Job drawing, mm, ordinate dimensions from the low corner. One solid piece. A direction names the side the tool comes from. Round coordinates to 2 decimals unless told otherwise and drop trailing zeros. Loops run counter-clockwise (first coordinate to the right, second up) from the corner with the lowest first, then second, coordinate; pieces in that order, holes last.
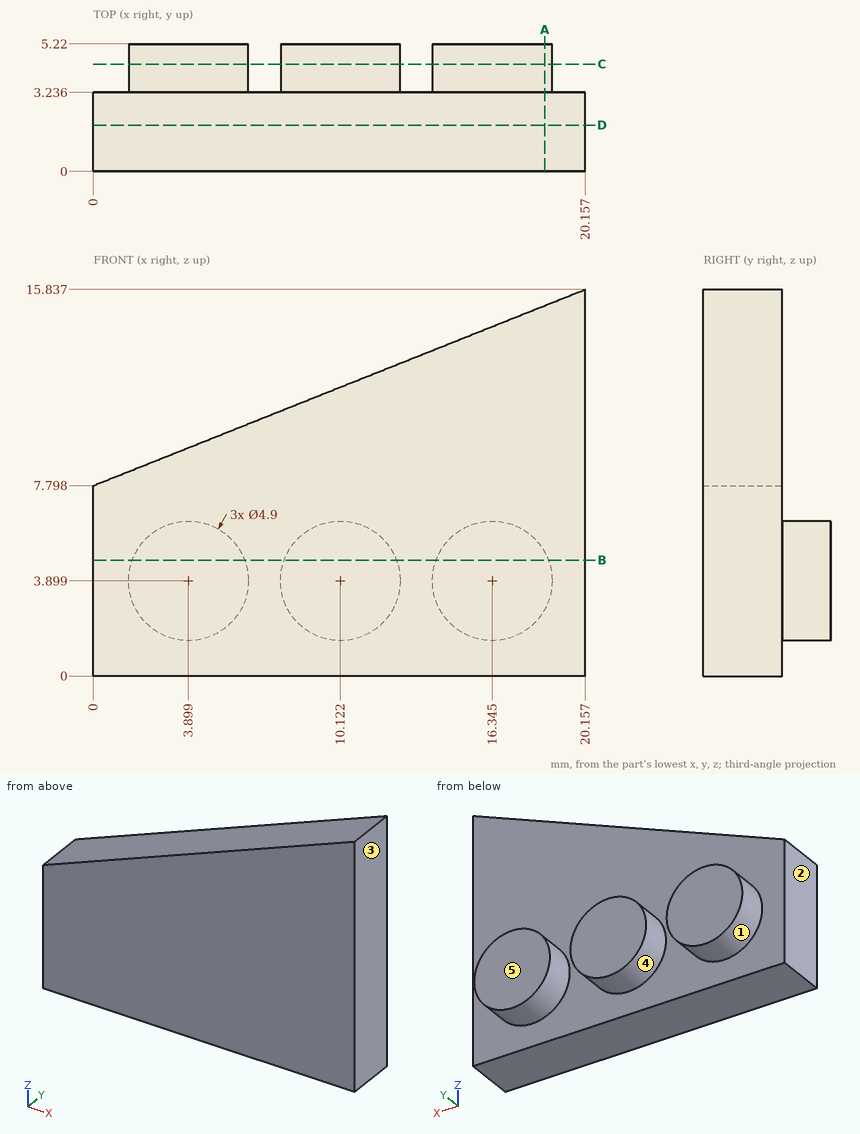
1) Slice it at A-A, the plane x = 18.5. Give the cut face in (y, z).
Values:
outline: (0, 0) - (3.24, 0) - (3.24, 2.73) - (5.22, 2.73) - (5.22, 5.06) - (3.24, 5.06) - (3.24, 15.18) - (0, 15.18) - close
2) Mould opens along X. For the marked faces 3, 4 and 5 say: released by +X, released by -X, zero draft, split by the parting line, or undercut.
Values:
face 3: released by +X
face 4: undercut
face 5: zero draft
3) Slice it at D-D, the plane y = 1.9. Give the cut face in (x, z), then the cut area to 3 significant figures.
Values:
outline: (0, 0) - (20.16, 0) - (20.16, 15.84) - (0, 7.8) - close
area: 238 mm2
4) Slice it at B-B, the plane z = 4.75. Give the cut face in (x, y) (1 decimal).
Values:
outline: (0, 0) - (20.2, 0) - (20.2, 3.2) - (18.6, 3.2) - (18.6, 5.2) - (14, 5.2) - (14, 3.2) - (12.4, 3.2) - (12.4, 5.2) - (7.8, 5.2) - (7.8, 3.2) - (6.2, 3.2) - (6.2, 5.2) - (1.6, 5.2) - (1.6, 3.2) - (0, 3.2) - close
5) Slice it at C-C, the plane y = 4.4. Give the number of separate pieces and of enclosed holes in the cut face.
Values:
separate pieces: 3
enclosed holes: 0
6) Tool access for the marked faces 1 and 2: list every direction of +Z, -Z, +X, -X, +Y, -Y with a clear straight run to the whole face (end or side of a thin tool).
Values:
face 1: +Y
face 2: +Z, -Z, -X, +Y, -Y
7) Wall check: line 1 along Y through (x, z) = (11.25, 10.5); line 2 along Z through (x, y) = (16.5, 4.1); line 3 along Z through (x, y) = (3, 2.2) (1 decimal). Give the ranges that are in metal, low to high.
Values:
line 1: y = 0 to 3.24
line 2: z = 1.45 to 6.34
line 3: z = 0 to 9
